The listing builds one solid part. Answer for the finished solid, in the listing's coordinates (mm). A direction names the side the tool comes from. Round coordinates to 2 decimals unless told otherwise and drop trailing zeros. Order: outer loops, then holes, each group sorted by start corner. A loop starts at its lowest first (then second) coordinate and runs counter-clockwise, first axis right, second up. Notation, with made-up numbers: (88.5, -22.75) - (132.5, -22.75) arc R26 cw to (132.5, 11.25) - close; hole circle Ø7 at (49.5, -3.75). An arc over 180 degrees is marked (long way). Write item = value, one per line.
from build123d import *

# Parameters (mm, degrees)
SKETCH_1_R          = 1.65
EXTRUDE_1_DEPTH     = 3
SKETCH_2_R          = 1.6
CUT_EXTRUDE_1_DEPTH = 15
CUT_EXTRUDE_2_DEPTH = 15
SKETCH_5_R          = 2.1
CUT_EXTRUDE_4_DEPTH = 10
EXTRUDE_2_DEPTH     = 3


with BuildPart() as part:
    # 草图1 → 凸台-拉伸1 (new body)
    with BuildSketch(Plane.XY):
        with BuildLine():
            Line((-10, -220), (10, -220))
            Line((10, -220), (22.697635701, -12.395491404))
            ThreePointArc((22.697635701, -12.395491404), (18.150671537, -5.407168438), (10.142345541, -7.726275101))
            ThreePointArc((10.142345541, -7.726275101), (0, -12.75), (-10.142345541, -7.726275101))
            ThreePointArc((-10.142345541, -7.726275101), (-18.150671537, -5.407168438), (-22.697635701, -12.395491404))
            Line((-22.697635701, -12.395491404), (-10, -220))
        make_face()
        with Locations((-11.313708499, -11.313708499)):
            Circle(SKETCH_1_R, mode=Mode.SUBTRACT)
        with Locations((0, -16)):
            Circle(SKETCH_1_R, mode=Mode.SUBTRACT)
        with Locations((11.313708499, -11.313708499)):
            Circle(SKETCH_1_R, mode=Mode.SUBTRACT)
    extrude(amount=EXTRUDE_1_DEPTH)

    # 草图2 → 切除-拉伸1 (cut)
    with BuildSketch(Plane.XY.offset(3)):
        with Locations((0, -216)):
            Circle(SKETCH_2_R)
        with Locations((0, -206)):
            Circle(SKETCH_2_R)
    extrude(amount=-CUT_EXTRUDE_1_DEPTH, mode=Mode.SUBTRACT)

    # 草图4 → 切除-拉伸2 (cut)
    with BuildSketch(Plane(origin=(0, 0, 0), x_dir=(-1, 0, 0), z_dir=(0, 0, -1))):
        with BuildLine():
            Line((-13.715926625, -28.201870805), (-10.113702702, -87.097711346))
            ThreePointArc((-10.113702702, -87.097711346), (-9.904103863, -88.030297779), (-9.411801117, -88.849618921))
            Line((-9.411801117, -88.849618921), (-2.292502811, -97.284018261))
            ThreePointArc((-2.292502811, -97.284018261), (0, -98.348965067), (2.292502811, -97.284018261))
            Line((2.292502811, -97.284018261), (9.411801117, -88.849618921))
            ThreePointArc((9.411801117, -88.849618921), (9.904103863, -88.030297779), (10.113702702, -87.097711346))
            Line((10.113702702, -87.097711346), (13.715926625, -28.201870805))
            ThreePointArc((13.715926625, -28.201870805), (12.496725506, -25.600326268), (9.649370007, -25.216852668))
            ThreePointArc((9.649370007, -25.216852668), (0, -27), (-9.649370007, -25.216852668))
            ThreePointArc((-9.649370007, -25.216852668), (-12.496725506, -25.600326268), (-13.715926625, -28.201870805))
        make_face()
    extrude(amount=-CUT_EXTRUDE_2_DEPTH, mode=Mode.SUBTRACT)

    # 草图5 → 切除-拉伸4 (cut)
    with BuildSketch(Plane.XY.offset(3)):
        with Locations((0, -188.402692504)):
            Circle(SKETCH_5_R)
        with Locations((0, -118.402692504)):
            Circle(SKETCH_5_R)
    extrude(amount=-CUT_EXTRUDE_4_DEPTH, mode=Mode.SUBTRACT)

    # 草图3 → 凸台-拉伸2 (add)
    with BuildSketch(Plane.XY.offset(3)):
        with BuildLine():
            Line((10, -220), (0, -220))
            Line((0, -220), (0, -221.563277065))
            ThreePointArc((0, -221.563277065), (4.306596315, -222.17357498), (8.274056276, -223.956408914))
            ThreePointArc((8.274056276, -223.956408914), (9.263696736, -224.000871181), (9.806001156, -223.171853056))
            Line((9.806001156, -223.171853056), (10, -220))
        make_face()
        with BuildLine():
            Line((0, -220), (-10, -220))
            Line((-10, -220), (-9.806001156, -223.171853056))
            ThreePointArc((-9.806001156, -223.171853056), (-9.263696736, -224.000871181), (-8.274056276, -223.956408914))
            ThreePointArc((-8.274056276, -223.956408914), (-4.306596315, -222.17357498), (0, -221.563277065))
            Line((0, -221.563277065), (0, -220))
        make_face()
    extrude(amount=-EXTRUDE_2_DEPTH)


solid = part.part
Q1. For faces 1 (the face through (5.9, -93.01, 1.48)), 2 (the face through (0, -113, 3)), determine the directions among +Z, -Z, +X, -X, +Y, -Y from which every point of the face is accessible in a straight line to the end or side of a thin tool.
Model answer:
face_1 = +Z, -Z
face_2 = +Z, +X, -X, +Y, -Y
Q2. Section C-C on y = -131 is taken. Determine the outline of the cut face in (x, z), then the cut area to 3 significant figures.
Model answer:
outline = (-15.44, 0) - (15.44, 0) - (15.44, 3) - (-15.44, 3) - close
area = 92.7 mm^2
Q3. Determine the mould class of faces 3 (the face through (0, -113, 0)), 4 (the face through (-11.89, -58.06, 1.48)), 5 (the face through (0.16, -12.75, 1.48)) for opening direction X: released by +X, released by -X, zero draft, split by the parting line, or undercut.
Model answer:
face_3 = zero draft
face_4 = undercut
face_5 = undercut
Q4. Find the intervals of material crossed by line 1 (X direction, y = -88, z = 2.3); line 2 (Y direction, x = 5, z = 1.25); line 3 (X direction, y = -57, z = 0.65), in increasing order. Write a range as from..to.
Model answer:
line_1 = -18.07..-9.92, 9.92..18.07
line_2 = -222.39..-94.08, -26.53..-11.73
line_3 = -19.97..-11.95, 11.95..19.97
Q5. Section B-B on z = 2.25 is taken. Count the separate pieces of the cut face and the enclosed holes in it, then the cut area to 3 significant figures.
Model answer:
separate_pieces = 1
enclosed_holes = 8
area = 5,350 mm^2
Q6. A flat-ended cylindrical pin translates along its axis: P1, Ø1, axis at x = 8, z = 0.5, coming from the -Y side. Find the tip coordinate at first contact, or state that the pin passes through.
Model answer:
P1 = -224.06
Q7. Section A-A on y = -40 is taken. Determine the outline of the cut face in (x, z), then the cut area to 3 significant figures.
Model answer:
outline = (-21.01, 0) - (-12.99, 0) - (-12.99, 3) - (-21.01, 3) - close; (12.99, 0) - (21.01, 0) - (21.01, 3) - (12.99, 3) - close
area = 48.1 mm^2
Q8. Section D-D on x = -18.5 is taken. Determine the outline of the cut face in (y, z).
Model answer:
outline = (-81.03, 0) - (-5.55, 0) - (-5.55, 3) - (-81.03, 3) - close
